Input: part model. Units: mm. Frame: model coordinates. Round coordinates to 2 decimals unless told otherwise and drop trailing zeros. Loops run counter-clockwise (first coordinate to the right, second up) from the corner with the lowest first, then second, coordinate; pieces in that order, holes last.
1) Section B-B, the plane y = 28. Return loops of the section in (x, z), and give its area (3 significant figures).
2) Ray query, line 1 along Y through (x, z) = (53, 659); line 2 along Y through (x, z) = (137, 486). Return the intervals inside material, ascending.
3) Section A-A, the plane z = 989. Return loops of the section in (x, y), and give its area (3 significant figures).
4) First-contact query: pin 1 (9 mm diameter, centred on x = 34.5, y = 54.5, fed in from +Z); pin 2 (9 mm diameter, centred on x = 30, y = 57.5, fed in from -Z); pin 3 (1 mm diameter, centred on x = 103, z = 520, fed in from -Y); pin 4 (2 mm diameter, centred on x = 80, y = 44, fed in from -Z). Flat tips, straight axial feed; report the tip coordinate or a pass-through.
from build123d import *

# Parameters (mm, degrees)
BOSS_EXTRUDE1_DEPTH = 1231.392
SKETCH5_R           = 22.225
SKETCH5_W           = 28.575
SKETCH5_H           = 50.8
CUT_EXTRUDE2_DEPTH  = 1252.786284181
FILLET1_R           = 6.35


with BuildPart() as part:
    # Sketch1 → Boss-Extrude1 (new body)
    with BuildSketch(Plane.XY):
        Polygon((232.654542571, 12.267259413), (25.64456355, 67.73541462), (22.35756176, 55.468156604), (229.367540781, 1.397e-06), align=None)
    extrude(amount=BOSS_EXTRUDE1_DEPTH)

    # Sketch5 → Cut-Extrude2 (cut, through all)
    with BuildSketch(Plane(origin=(18.651713196, 69.609143174, 0), x_dir=(0.9659258280351158, -0.25881903858618227, 0), z_dir=(0.2588190385861823, 0.965925828035116, 0))):
        with Locations((7.239531392, -721.8045)):
            Circle(SKETCH5_R)
        with Locations((7.239531392, -240.792)):
            Circle(SKETCH5_R)
        with Locations((21.527031392, -1205.992)):
            Rectangle(SKETCH5_W, SKETCH5_H)
        with Locations((21.527031392, -25.4)):
            Rectangle(SKETCH5_W, SKETCH5_H)
    extrude(amount=-CUT_EXTRUDE2_DEPTH, mode=Mode.SUBTRACT)

    # Fillet1
    fillet1_edges = [part.edges().sort_by_distance(p)[0] for p in [
        (51.602393192, 54.206031584, 1180.592),
        (51.602393192, 54.206031584, 50.8),
    ]]
    fillet(fillet1_edges, radius=FILLET1_R)


solid = part.part
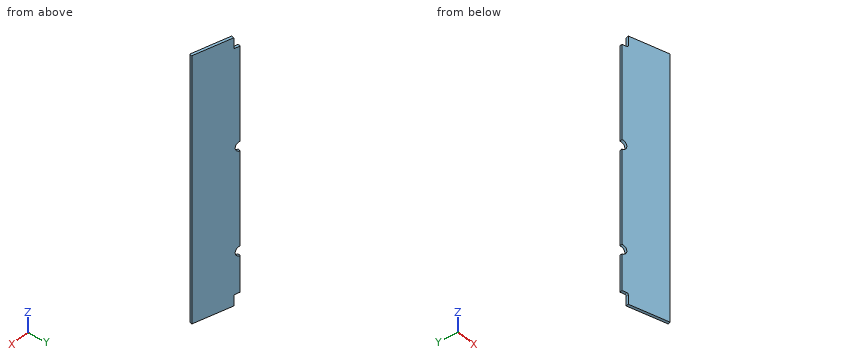
Final values:
1. outline: (124.87, 0) - (173.94, 0) - (173.94, 1231.39) - (124.87, 1231.39) - close
1. area: 60,400 mm2
2. line 1: y = 47.26 to 60.41
2. line 2: y = 24.75 to 37.9
3. outline: (22.36, 55.47) - (229.37, 0) - (232.65, 12.27) - (25.64, 67.74) - close
3. area: 2,720 mm2
4. pin 1: stops at z = 1180.59
4. pin 2: stops at z = 50.8
4. pin 3: stops at y = 33.73
4. pin 4: stops at z = 0
